Input: part model. Units: mm. Frame: model coordinates. A direction names the side the tool comes from. Coordinates: 2 decimals unless noted, no trailing zeros. Order: outer loops, then holes, each group sorted by start corner. A loop starts at its lowest first (then second) coordinate and runs counter-clockwise, first axis right, second up. Notation, with made-up numbers: (-6, -15) - (10, -15) arc R33 ccw to (10, 14) - close; hole circle Ø6 at (59, -11). An arc over 180 degrees is marked (long way). Use a Markdown table: item, result. Add a question column.
from build123d import *

# Parameters (mm, degrees)
F1_DEPTH = 293
F2_W     = 35
F2_H     = 35
F2_R     = 4
F3_DEPTH = 5
F4_W     = 40
F4_H     = 40
F4_R     = 4
F5_DEPTH = 5


with BuildPart() as f1:
    # F0 (on Right) → F1 (new body)
    with BuildSketch(Plane.YZ):
        Polygon((-7.9736986477, 15.6249996814), (-7.9736986477, -24.3750003186), (-2.9736986477, -24.3750003186), (-2.9736986477, 10.6249996814), (32.0263013523, 10.6249996814), (32.0263013523, 15.6249996814), align=None)
    extrude(amount=F1_DEPTH)

    # F2 (on face) → F3 (join)
    with BuildSketch(Plane.YZ.offset(293)):
        Polygon((-7.9736986477, 15.6249996814), (-7.9736986477, -24.3750003186), (-2.9736986477, -24.3750003186), (-2.9736986477, 10.6249996814), (32.0263013523, 10.6249996814), (32.0263013523, 15.6249996814), align=None)
        with Locations((14.5263013523, -6.8750003186)):
            Rectangle(F2_W, F2_H)
        with Locations((12.0263013523, -4.3750003186)):
            Circle(F2_R, mode=Mode.SUBTRACT)
    extrude(amount=F3_DEPTH)

    # F4 (on face) → F5 (join)
    with BuildSketch(Plane(origin=(0, 0, 0), x_dir=(0, -1, 0), z_dir=(-1, 0, 0))):
        with Locations((-12.0263013523, -4.3750003186)):
            Rectangle(F4_W, F4_H)
        with Locations((-12.0263013523, -4.3750003186)):
            Circle(F4_R, mode=Mode.SUBTRACT)
    extrude(amount=F5_DEPTH)


solid = f1.part
1) Cut plane C-C (x = 256). Return the cut outline in (y, z) (3 decimals).
2) Cut plane A-A (y = 13.5). Return the cut outline in (x, z) (3 decimals).
3) Material intervals for L1, parallel to X at y = 20, z = 10; L2, parallel to Y at x = 153, z = -22; L3, parallel to Z at x = 129.5, y = 14 (3 decimals), sorted ascending.
4) Contact query for flat-ended pins moving along their axis: P1, Ø10.5, axis at x = 203, z = -3.5, coming from the +Y side; P2, Ø2, axis at x = 83.5, y = 11.5, coming from the -Z side (3 decimals). Output: stop coordinate, or through.
5) Pull-direction query (X, two-part tool) for faces 1 (the flat face through (-5, 17, -4)), 2 (the flat face through (144, 14, 10.625)), 3 (the flat face through (149, 12, 15.625)); classes: pulls with the +X half, pulls with the -X half, needs draft (parallel to the pull), parting line crosses it, or undercut.
6) Cut plane B-B (z = -20.5). Return the cut outline in (x, y).
7) Reachability of faces 4 (the flat face through (0, 15, -11)), 5 (the flat face through (181, 32.026, 12)) from +Z, -Z, +X, -X, +Y, -Y: full face, straight path, thin tool, end or side. Return the list, or none.
Computed:
| question | item | result |
|---|---|---|
| 1 | outline | (-7.974, -24.375) - (-2.974, -24.375) - (-2.974, 10.625) - (32.026, 10.625) - (32.026, 15.625) - (-7.974, 15.625) - close |
| 2 | outline | (-5, -24.375) - (0, -24.375) - (0, -8.094) - (-5, -8.094) - close; (-5, -0.656) - (0, -0.656) - (0, 10.625) - (293, 10.625) - (293, -0.656) - (298, -0.656) - (298, 15.625) - (-5, 15.625) - close; (293, -24.375) - (298, -24.375) - (298, -8.094) - (293, -8.094) - close |
| 3 | L1 | x = -5 to 0, 293 to 298 |
| 3 | L2 | y = -7.97 to -2.97 |
| 3 | L3 | z = 10.625 to 15.625 |
| 4 | P1 | stops at y = -2.97 |
| 4 | P2 | stops at z = 10.625 |
| 5 | face 1 | pulls with the -X half |
| 5 | face 2 | undercut |
| 5 | face 3 | needs draft |
| 6 | outline | (-5, -7.97) - (298, -7.97) - (298, 32.03) - (293, 32.03) - (293, -2.97) - (0, -2.97) - (0, 32.03) - (-5, 32.03) - close |
| 7 | face 4 | -Z, +Y |
| 7 | face 5 | +Z, -Z, +X, -X, +Y |
